Here's how the part is built. I have some questions about the finished solid (model axes, mm). A direction names the side the tool comes from. Round coordinates to 2 decimals unless told otherwise and drop trailing zeros. Write each loop counter-clockwise with the first axis right and the second up, starting at its lowest first coordinate (ties: lowest second). Pieces come first, ordered by that corner, then holes. Notation, with made-up numbers: (16, 8) -> (22, 8) arc R17 ccw to (22, 12) -> close; hole circle Ø4 at (71.25, -19.5). An arc over 180 degrees is marked (long way). Put each result on its own line as item: value. Start each with the question number.
1. Suppose I cut it at A-A (y = 4). Please give me the cut outline in (x, z).
2. I need wall thicknesses on probe 1 along X at (y, z) = (1, -109.5); probe 2 along Y at (x, z) = (-2.25, -35); probe 3 along X at (y, z) = (10.75, -174.5). Which ranges of each line are inside material? Lowest first, please. Write a range as from..to.
3. For pin 1 (2.5 mm diameter, centred on y = 4, z = -92, fed in from -X); pin 2 (1.1 mm diameter, centred on x = -2, z = -73, fed in from +Y); pin 3 (4 mm diameter, centred on y = 15.5, z = -155.5, fed in from +X); pin 4 (12 mm diameter, centred on y = 13.5, z = -91, fed in from -X), each with a flat end and sliding along its axis, tell me the tip position at first contact or that it passes through.
4. Which directions (+Z, -Z, +X, -X, +Y, -Y) give clear straight access to the entire face, cutting with the end or side of a thin tool? Please do faces 1 (the face through (-4.152, 5.599, -109.569)), 2 (the face through (0, 5, -110)), 3 (the face through (-7.842, 18, -110)).
5. We'd pull the mould along Y, two halves only. Please class faces 4 (the face through (-6, 22.225, -110)), 5 (the face through (-5, 21.336, -110)), 6 (the face through (-4.9, 5.1, -109.6)), 7 (the face through (-0.889, 5, -110)): +Y half, -Y half, draft (parallel to the pull), parting line (faces both ways), or undercut.
```python
from build123d import *

# Parameters (mm, degrees)
BOSS_EXTRUDE1_DEPTH = 222.25
FILLET1_R           = 0.889


with BuildPart() as part:
    # Sketch1 → Boss-Extrude1 (new body)
    with BuildSketch(Plane.XY):
        with BuildLine():
            Line((0, 8.73125), (0, 0))
            Line((0, 0), (-3.96875, 0))
            ThreePointArc((-3.96875, 0), (-4.748467779, 4.757288038), (-7.604139417, 8.641215018))
            ThreePointArc((-7.604139417, 8.641215018), (-8.73125, 11.067482509), (-7.604139417, 13.49375))
            Line((-7.604139417, 13.49375), (-8.73125, 13.49375))
            Line((-8.73125, 13.49375), (-8.73125, 22.225))
            Line((-8.73125, 22.225), (-3.175, 22.225))
            Line((-3.175, 22.225), (-3.175, 21.336))
            Line((-3.175, 21.336), (-7.84225, 21.336))
            Line((-7.84225, 21.336), (-7.84225, 14.38275))
            Line((-7.84225, 14.38275), (-7.604139417, 14.38275))
            ThreePointArc((-7.604139417, 14.38275), (-6.769194058, 13.799015865), (-7.03073038, 12.814395103))
            ThreePointArc((-7.03073038, 12.814395103), (-7.84225, 11.067482509), (-7.03073038, 9.320569916))
            ThreePointArc((-7.03073038, 9.320569916), (-4.123486495, 5.538022334), (-3.052821022, 0.889))
            Line((-3.052821022, 0.889), (-0.889, 0.889))
            Line((-0.889, 0.889), (-0.889, 8.73125))
            Line((-0.889, 8.73125), (0, 8.73125))
        make_face()
    extrude(amount=-BOSS_EXTRUDE1_DEPTH)

    # Fillet1
    fillet1_edges = [part.edges().sort_by_distance(p)[0] for p in [
        (0, 0, -111.125),
        (-3.96875, 0, -111.125),
        (-8.73125, 13.49375, -111.125),
        (-8.73125, 22.225, -111.125),
    ]]
    fillet(fillet1_edges, radius=FILLET1_R)


solid = part.part
```
Verdict:
1. outline: (-4.46, -222.25) -> (-3.53, -222.25) -> (-3.53, 0) -> (-4.46, 0) -> close; (-0.89, -222.25) -> (0, -222.25) -> (0, 0) -> (-0.89, 0) -> close
2. probe 1: x = -3.94..-3.05, -0.89..0
2. probe 2: y = 0..0.89
2. probe 3: x = -8.72..-7.82
3. pin 1: stops at x = -4.97
3. pin 2: stops at y = 0.89
3. pin 3: stops at x = -6.72
3. pin 4: stops at x = -8.73
4. face 1: +Z, -Z
4. face 2: +Z, -Z, +X, +Y, -Y
4. face 3: +Z, -Z, +X
5. face 4: +Y half
5. face 5: undercut
5. face 6: -Y half
5. face 7: draft
